The listing builds one solid part. Answer for the finished solid, in the listing's coordinates (mm). A direction names the side the tool comes from. Give positions to 0.01 mm unless a question says otherwise; leave off trailing zeros. Order: outer loops, then holes, each group sorted by start corner. A loop starts at its lowest first (then second) coordinate and runs counter-clockwise, first axis right, second up. Notation, with made-up numbers: (30.25, -36.5) - (65.25, -36.5) arc R11 ccw to (65.25, -18.5) - close; hole circle Ø9 at (66, 62). An arc over 180 degrees is marked (long way). Answer as CSV lines item,"result". Start each with the question number.
1. Which of the six approach directions +Z, -Z, +X, -X, +Y, -Y give full straight-line access (tool end or side, diameter ignored) to faces 1 (the flat face through (12, 20, 5)), 2 (the flat face through (-66, 13, 0)), 3 (the flat face through (-40, 10, -15)), 4 (the flat face through (-40, 10, 15))?
2. Section D-D on x = -24.5 is taken. Give the vertices of the cut face in (y, z).
3. Consider line 1 along X through (y, z) = (10, 0); line 2 along X through (y, z) = (30.5, 0); line 3 along Z through (x, y) = (-35, 13). Determine where each line is inside the solid, lowest interval first. Write a range as [from, to].
4. Determine the mould class of faces 5 (the cylindrical face through (-66.24, 6.41, -0.33)), 6 (the flat face through (-41.188, 4.93, 22.516)), 7 (the cylindrical face through (-13.73, 20.28, -0.48)), 8 (the flat face through (-81.238, 6, -20)) for opening direction Z: +Z half, -Z half, draft (parallel to the pull), parting line (faces both ways), or undercut.
5. Flat-ended cylindrical pins translate along their axes: pin 1 (6 mm diameter, centred on y = 16.5, z = 13, fed in from +X); pin 2 (20 mm diameter, centred on x = -1.24, z = 0, fed in from +Y); pin 3 (10 mm diameter, centred on x = -54, z = 15, fed in from +Y); pin 4 (5 mm diameter, centred on y = 14, z = -1, fed in from -X). Find the tip coordinate at first contact, or state that the pin passes through.
6. Section B-B on y = 34.5 is taken. Give the vertices of the cut face in (x, z).
7. Section C-C on x = 4.5 is taken. Give the vertices of the cut face in (y, z), and give its area (3 significant figures).
8. Section A-A on z = 0 is taken. Give the vertices of the cut face in (x, y), and give its area (3 significant figures).
from build123d import *

# Parameters (mm, degrees)
EXTRUDE_3_DEPTH          = 10
EXTRUDE_7_DEPTH          = 3
CUT_EXTRUDE_3_DEPTH      = 86.986132552
CUT_EXTRUDE_3_DEPTH_BACK = 86.986132552
SKETCH_7_R               = 20
EXTRUDE_8_DEPTH          = 30
RIB_START                = -5
RIB_1_DEPTH              = 10
SKETCH_10_R              = 12.5
CUT_EXTRUDE_4_DEPTH      = 94.939421923
SKETCH_11_W              = 15.5
SKETCH_11_H              = 10
CUT_EXTRUDE_5_DEPTH      = 94.939421923


# Read off the part's stored shape, not the designer's step: 筋1
with BuildPart() as part:
    # 草图1 → 凸台-拉伸3 (new body)
    with BuildSketch(Plane(origin=(0, 0, 0), x_dir=(1, 0, 0), z_dir=(0, 1, 0))):
        with BuildLine():
            Line((-81.238014447, 25), (-81.238014447, -25))
            Line((-81.238014447, -25), (0, -19.96164623))
            ThreePointArc((0, -19.96164623), (18.761985553, 0), (0, 19.96164623))
            Line((0, 19.96164623), (-81.238014447, 25))
        make_face()
    extrude(amount=EXTRUDE_3_DEPTH)

    # 草图2 → 凸台-拉伸7 (add)
    with BuildSketch(Plane(origin=(0, 10, 0), x_dir=(1, 0, 0), z_dir=(0, 1, 0))):
        with BuildLine():
            Line((-81.238014447, 25), (-81.238014447, -25))
            ThreePointArc((-81.238014447, -25), (-56.238014447, 0), (-81.238014447, 25))
        make_face()
    extrude(amount=EXTRUDE_7_DEPTH)

    # 草图5 → 切除-拉伸3 (cut, two sides: drawn at the far end of the back side and taken through both)
    with BuildSketch(Plane(origin=(0, 13, 0), x_dir=(1, 0, 0), z_dir=(0, 1, 0)).offset(-CUT_EXTRUDE_3_DEPTH_BACK)):
        with BuildLine():
            Line((-306.644606732, 15), (-81.238014447, 15))
            ThreePointArc((-81.238014447, 15), (-66.238014447, 0), (-81.238014447, -15))
            Line((-81.238014447, -15), (-306.644606732, -15))
            Line((-306.644606732, -15), (-757.457791303, -15))
            Line((-757.457791303, -15), (-757.457791303, 15))
            Line((-757.457791303, 15), (-306.644606732, 15))
        make_face()
    extrude(amount=CUT_EXTRUDE_3_DEPTH + CUT_EXTRUDE_3_DEPTH_BACK, mode=Mode.SUBTRACT)

    # 草图7 → 凸台-拉伸8 (add)
    with BuildSketch(Plane(origin=(0, 10, 0), x_dir=(1, 0, 0), z_dir=(0, 1, 0))):
        with Locations(Location((-1.238014447, 0, 0), (0, 0, 86.451080997))):
            Circle(SKETCH_7_R)
    extrude(amount=EXTRUDE_8_DEPTH)

    # 筋1 outline → 筋1 (add)
    with BuildSketch(Plane.XY.offset(RIB_START)):
        Polygon((-51.238014447, 13), (-58, 13), (-58, 10), (-19, 10), (-19, 31.268208187), (-20.602931178, 30.359880519), align=None)
    extrude(amount=RIB_1_DEPTH)

    # 草图10 → 切除-拉伸4 (cut, through all)
    with BuildSketch(Plane(origin=(0, 40, 0), x_dir=(1, 0, 0), z_dir=(0, 1, 0))):
        with Locations(Location((-1.238014447, 0, 0), (0, 0, 270))):
            Circle(SKETCH_10_R)
    extrude(amount=-CUT_EXTRUDE_4_DEPTH, mode=Mode.SUBTRACT)

    # 草图11 → 切除-拉伸5 (cut, through all)
    with BuildSketch(Plane(origin=(0, 40, 0), x_dir=(1, 0, 0), z_dir=(0, 1, 0))):
        with Locations((6.511985553, 0)):
            Rectangle(SKETCH_11_W, SKETCH_11_H)
    extrude(amount=-CUT_EXTRUDE_5_DEPTH, mode=Mode.SUBTRACT)


solid = part.part
Checks:
1,face 1,"+Y, -Y"
1,face 2,"+Z, -Z, -X, +Y"
1,face 3,"-Z, +Y"
1,face 4,"+Z, +Y"
2,outline,"(0, -21.48) - (10, -21.48) - (10, -5) - (28.15, -5) - (28.15, 5) - (10, 5) - (10, 21.48) - (0, 21.48) - close"
3,line 1,"x = [-66.24, -13.74], [14.26, 18.76]"
3,line 2,"x = [-21.24, -13.74], [14.26, 18.76]"
3,line 3,"z = [-5, 5]"
4,face 5,"undercut"
4,face 6,"+Z half"
4,face 7,"undercut"
4,face 8,"draft"
5,pin 1,"stops at x = 16.08"
5,pin 2,"passes through"
5,pin 3,"stops at y = 10"
5,pin 4,"stops at x = -66.6"
6,outline,"circle Ø40 at (-1.24, 0); hole (10.22, -5) - (14.26, -5) - (14.26, 5) - (10.22, 5) arc R12.5 ccw (long way) to start"
7,outline,"(0, -19.16) - (40, -19.16) - (40, -11.11) - (0, -11.11) - close; (0, 11.11) - (40, 11.11) - (40, 19.16) - (0, 19.16) - close"
7,area,"644 mm²"
8,outline,"(-66.24, 0) - (-13.74, 0) - (-13.74, 40) - (-21.24, 40) - (-21.24, 30) - (-51.24, 13) - (-66.24, 13) - close; (14.26, 0) - (18.76, 0) - (18.76, 40) - (14.26, 40) - close"
8,area,"1,320 mm²"
